Input: dimensioned drawing with shaded views. Units: mm. Origin: part minimum x, y, z. A direction names the side the tool comes from. Give positions to 0.01 mm unless a question says otherwise; leave off trailing zeros. Write each loop counter-clockwise with the first axis right and the second up, starting at its lowest first coordinate (ties: lowest second). Pieces come first, ordered by that corner, then holes. Notation, with made-up numbers: (14.25, -20.75) -> (51.25, -20.75) arc R19 cw to (51.25, 10.25) -> close; hole circle Ø8 at (20.5, 36.5). An arc over 180 degrees is marked (long way). Answer as a JSON object with one key per item and string values. Group by question number.
(1) Set-up query: the marked faces 1, 2, 3 and 4. Return all of +Z, -Z, +X, -X, +Y, -Y with unobstructed straight access to the full face (end or side cutting, diameter ignored); none if empty.
(2) Section query D-D on y = 51.5. Output: boundary loops of the cut face in (x, z).
(3) Section query C-C on z = 8. Output: boundary loops of the cut face in (x, y), plus the area to 4 significant figures.
(4) Material intervals for probe 1 along Z at (x, y) = (32.25, 51.5); probe 2 along Z at (x, y) = (1.8, 17.1); probe 3 along Y at (x, z) = (31, 12), sorted ascending.
(5) Section query B-B on z = 21. Output: boundary loops of the cut face in (x, y).
(6) Draft query along X for the marked faces 5, 6, 7 and 8. Return one class per face: +X half, -X half, draft (parallel to the pull), parting line (faces both ways), or undercut.
(7) Contact query for flat-ended pins moving along their axis: pin 1 Ø1.8 at (y, z) = (51.5, 8) entering from +X; pin 2 Ø3 at (x, y) = (21, 9) entering from +Z; pin 3 Ø2 at (x, z) = (5.5, 19) entering from +Y. Output: stop coordinate, or through.
(8) Section query A-A on y = 37.4. Output: boundary loops of the cut face in (x, z), plus the area to 3 significant figures.
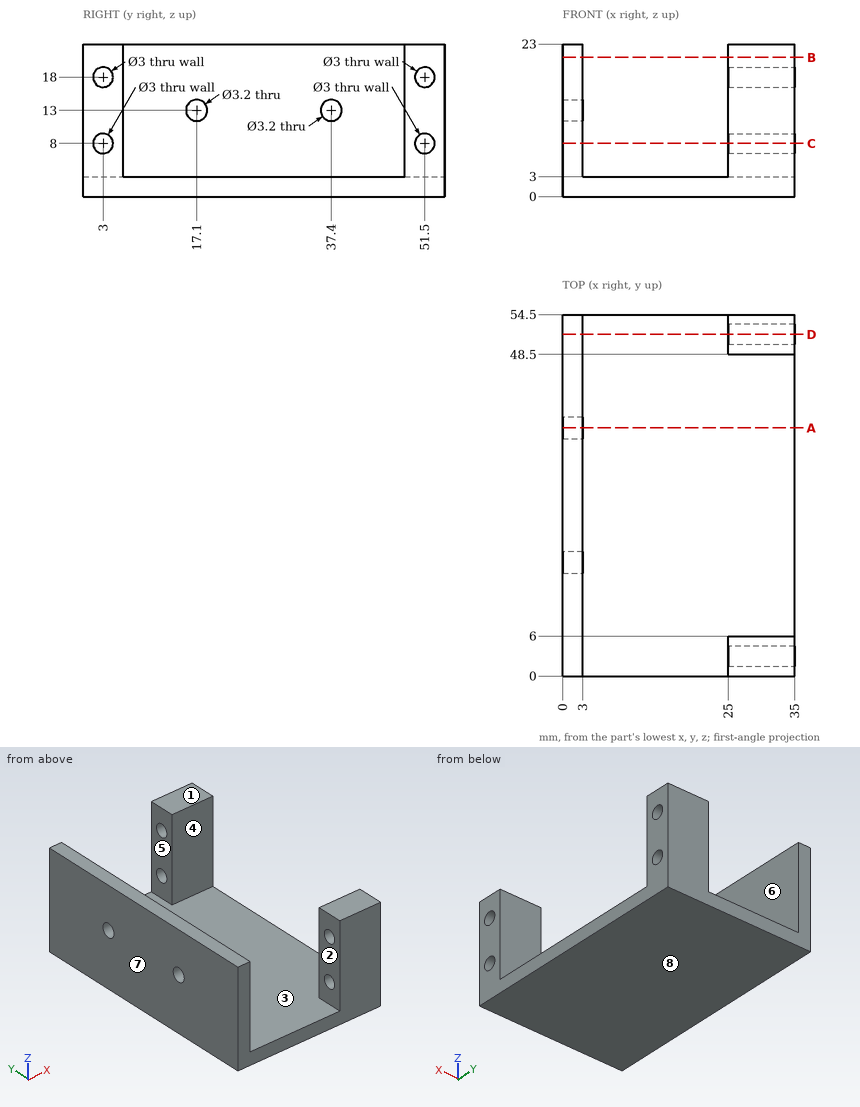
Answer list:
{
 "1": {"face 1": "+Z, +X, -X, +Y, -Y", "face 2": "+Z, +Y, -Y", "face 3": "+Z", "face 4": "+Z, +X"},
 "2": {"outline": "(0, 0) -> (35, 0) -> (35, 6.5) -> (25, 6.5) -> (25, 3) -> (3, 3) -> (3, 23) -> (0, 23) -> close; (25, 9.5) -> (35, 9.5) -> (35, 16.5) -> (25, 16.5) -> close; (25, 19.5) -> (35, 19.5) -> (35, 23) -> (25, 23) -> close"},
 "3": {"outline": "(0, 0) -> (3, 0) -> (3, 54.5) -> (0, 54.5) -> close; (25, 0) -> (35, 0) -> (35, 1.5) -> (25, 1.5) -> close; (25, 4.5) -> (35, 4.5) -> (35, 6) -> (25, 6) -> close; (25, 48.5) -> (35, 48.5) -> (35, 50) -> (25, 50) -> close; (25, 53) -> (35, 53) -> (35, 54.5) -> (25, 54.5) -> close", "area": "223.5 mm2"},
 "4": {"probe 1": "0 to 6.5, 9.5 to 16.5, 19.5 to 23", "probe 2": "0 to 11.4, 14.6 to 23", "probe 3": "0 to 6, 48.5 to 54.5"},
 "5": {"outline": "(0, 0) -> (3, 0) -> (3, 54.5) -> (0, 54.5) -> close; (25, 0) -> (35, 0) -> (35, 6) -> (25, 6) -> close; (25, 48.5) -> (35, 48.5) -> (35, 54.5) -> (25, 54.5) -> close"},
 "6": {"face 5": "undercut", "face 6": "undercut", "face 7": "-X half", "face 8": "draft"},
 "7": {"pin 1": "x = 3", "pin 2": "z = 3", "pin 3": "through"},
 "8": {"outline": "(0, 0) -> (35, 0) -> (35, 3) -> (3, 3) -> (3, 11.4) -> (0, 11.4) -> close; (0, 14.6) -> (3, 14.6) -> (3, 23) -> (0, 23) -> close", "area": "155 mm2"}
}
